For this review, use the dimensioned drawing (mm, ordinates from the lowest corner) and the shaded views. Coordinates: 2 decimals unless noted, no trailing zeros. Loops run counter-clockwise (first coordinate to the right, second up) from the corner with the lowest first, then second, coordinate; pieces in that order, holes last. Notation, with made-up numbers: (83, -2) - (105, -2) arc R20 cw to (105, 32) - close; hole circle Ø2 at (-33.5, 24). An arc over 180 degrees is marked (long way). Use one line per item in the form item = value. Start each with the question number.
(1) Add section C-C (y = 1.25). State the section outline as (x, z) points, plus the area to 3 significant figures.
(2) Clearance check with flat-ended pins moving along their axes: pin 1 Ø4 at (x, y) = (19, 7) entering from -Z; pin 2 Ø2 at (x, z) = (20, 78.5) entering from +Y. State where each tip first meets the part, or that it passes through.
(3) For L1, parallel to Z at x = 20, y = 2; L2, parallel to X at y = 3.1, z = 77; L3, parallel to Z at x = 18, y = 5.25 (1 decimal), list the stretches that pass through material, from the lowest coordinate up.
(4) Add section B-B (x = 20). State the section outline as (y, z) points, plus the area to 3 significant figures.
(5) The part is to be moulded in two halves that separate along Z. For the marked faces 1, 2 and 3, say which applies: pulls with the +Z half, pulls with the -Z half, needs draft (parallel to the pull), parting line crosses it, or undercut.
(6) Add section D-D (x = 4). State the section outline as (y, z) points.
(7) Add section A-A (y = 7). State the section outline as (x, z) points.
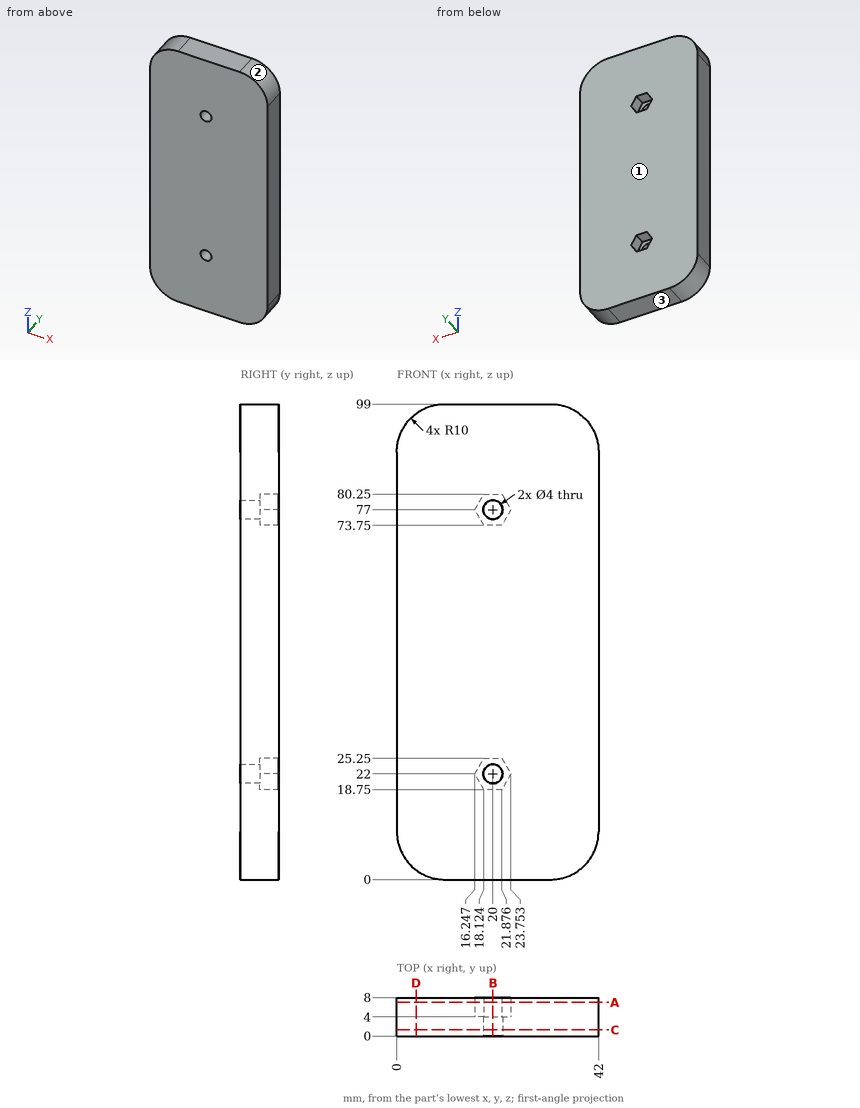
Computed values:
q1.outline = (0, 10) arc R10 ccw to (10, 0) - (32, 0) arc R10 ccw to (42, 10) - (42, 89) arc R10 ccw to (32, 99) - (10, 99) arc R10 ccw to (0, 89) - close; hole circle Ø4 at (20, 22); hole circle Ø4 at (20, 77)
q1.area = 4,050 mm^2
q2.pin_1 = 0
q2.pin_2 = 4
q3.L1 = 0 to 20, 24 to 75, 79 to 99
q3.L2 = 0 to 18, 22 to 42
q3.L3 = 0 to 19, 25 to 74, 80 to 99
q4.outline = (0, 0) - (8, 0) - (8, 18.75) - (4, 18.75) - (4, 20) - (0, 20) - close; (0, 24) - (4, 24) - (4, 25.25) - (8, 25.25) - (8, 73.75) - (4, 73.75) - (4, 75) - (0, 75) - close; (0, 79) - (4, 79) - (4, 80.25) - (8, 80.25) - (8, 99) - (0, 99) - close
q4.area = 708 mm^2
q5.face_1 = needs draft
q5.face_2 = pulls with the +Z half
q5.face_3 = pulls with the -Z half
q6.outline = (0, 2) - (8, 2) - (8, 97) - (0, 97) - close
q7.outline = (0, 10) arc R10 ccw to (10, 0) - (32, 0) arc R10 ccw to (42, 10) - (42, 89) arc R10 ccw to (32, 99) - (10, 99) arc R10 ccw to (0, 89) - close; hole (16.25, 22) - (18.12, 18.75) - (21.88, 18.75) - (23.75, 22) - (21.88, 25.25) - (18.12, 25.25) - close; hole (16.25, 77) - (18.12, 73.75) - (21.88, 73.75) - (23.75, 77) - (21.88, 80.25) - (18.12, 80.25) - close
